For this review, take the finished solid that the model builds, in its own axes (mm). A direction names the side the tool comes from. Give positions to 0.01 mm unless a question says otherwise; leave off trailing zeros. Loops run counter-clockwise (first coordinate to the right, second up) from the corner with the lowest first, then second, coordinate; pieces in that order, holes last.
Autodesk Inventor part; units mm, degrees
ref_plane "YZ Plane" through (0, 0, 0) normal (1, 0, 0) x (0, 1, 0)
ref_plane "XZ Plane" through (0, 0, 0) normal (0, 1, 0) x (-1, 0, 0)
ref_plane "XY Plane" through (0, 0, 0) normal (0, 0, 1) x (1, 0, 0)
sketch "Sketch1" plane through (0, 0, 0) normal (0, 0, 1) x (1, 0, 0)
  circle A0 centre (0, 0) radius 11.5
  arc A1 (20, 0) -> (-20, 0) centre (0, 0) ccw
  line L0 (20, 0) -> (20, -30)
  line L1 (-20, -30) -> (-20, 0)
  line L2 (35, -30) -> (35, -51)
  line L3 (35, -51) -> (-35, -51)
  line L4 (-35, -51) -> (-35, -30)
  line L5 (-35, -30) -> (-20, -30)
  line L6 (20, -30) -> (35, -30)
extrude "Extrusion1" add sketch "Sketch1" along normal blind 6
sketch "Sketch2" plane through (-35, -51, 0) normal (0, -1, 0) x (1, 0, 0)
  line L0 (30, 12) -> (30, -6)
  line L1 (30, -6) -> (40, -6)
  line L2 (40, -6) -> (40, 12)
  line L3 (40, 12) -> (30, 12)
  line L4 (30, 12) -> (40, -6) construction
  line L5 (30, -6) -> (40, 12) construction
  point P0 (35, 0)
  point P1 (35, 3)
  dimension "d7" = 18
  dimension "d8" = 10
extrude "Extrusion2" add sketch "Sketch2" against normal blind 20
fillet "Fillet1" radius 2 6 edges at (5, -41, 6) (-5, -41, 6) (5, -41, 0) (-5, -41, 0) (0, -31, 0) (0, -31, 6)
fillet "Fillet2" radius 4 2 edges at (0, -31, 12) (0, -31, -6)
fillet "Fillet3" radius 4 2 edges at (-35, -30, 3) (35, -30, 3)
sketch "Sketch3" plane through (0, 0, 6) normal (0, 0, 1) x (1, 0, 0)
  arc A0 (7.9976, -11.4908) -> (-7.9976, -11.4908) centre (0, 0) ccw
  arc A1 (7.9976, -16.682) -> (-7.9976, -16.682) centre (0, 0) ccw
  line L0 (4, -12.8417) -> (-4, -19.4934) construction
  line L1 (-4, -12.8417) -> (4, -19.4934) construction
  line L2 (-7.9976, -11.4908) -> (-7.9976, -16.682)
  line L3 (7.9976, -11.4908) -> (7.9976, -16.682)
  point P0 (0, -16.1675)
extrude "Extrusion3" cut sketch "Sketch3" against normal blind 10
sketch "Sketch4" plane through (0, 0, 6) normal (0, 0, 1) x (1, 0, 0)
  line L0 (-7.9976, -11.4908) -> (-7.9976, -16.682)
  line L1 (-7.9976, -16.682) -> (-19.8959, -16.682)
  arc A0 (7.9976, -16.682) -> (-7.9976, -16.682) centre (0, 0) ccw
  line L2 (7.9976, -16.682) -> (20, -16.682)
  line L3 (20, -30) -> (20, 0)
  line L4 (-7.9976, -16.682) -> (-17.0011, 1.4894)
  line L5 (-17.0011, 1.4894) -> (-8.7801, 14.2319)
  line L6 (-8.7801, 14.2319) -> (1.2495, 15.1362)
  line L7 (1.2495, 15.1362) -> (10.7036, 12.5877)
  line L8 (10.7036, 12.5877) -> (15.6744, 3.4985)
  line L9 (15.6744, 3.4985) -> (15.6744, -3.8181)
  line L10 (15.6744, -3.8181) -> (10.5163, -11.3974)
  line L11 (10.5163, -11.3974) -> (8.7045, -14.0594)
  line L12 (8.7045, -14.0594) -> (7.9976, -16.682)
  line L13 (-19.8959, -16.682) -> (-31.3329, 15.1362)
  line L14 (-31.3329, 15.1362) -> (-3.7653, 25.0453)
  line L15 (-3.7653, 25.0453) -> (28.3359, 16.3269)
  line L16 (28.3359, 16.3269) -> (26.8111, -11.3974)
  line L17 (26.8111, -11.3974) -> (20, -16.682)
extrude "Extrusion4" cut sketch "Sketch4" against normal blind 10
sketch "Sketch5" plane through (-19.8959, -16.682, 6) normal (0, 1, 0) x (1, 0, 0)
  line L0 (-7.0101, -7.2709) -> (2.851, -7.2709)
  line L1 (2.851, -7.2709) -> (2.851, 8.3942)
  line L2 (2.851, 8.3942) -> (-7.0101, 8.3942)
  line L3 (-7.0101, 8.3942) -> (-7.0101, -7.2709)
  point P0 (19.8959, 6)
extrude "Extrusion5" cut sketch "Sketch5" along normal blind 10
fillet "Fillet4" radius 10 2 edges at (-20, -16.682, 3) (20, -16.682, 3)
properties part number "Secondary mount"
Q1. Mouldability with a two-part tool opening along Y and no side actions: class faces 6 (the flat face through (25, -30, 3)), 7 (the flat face through (0, -43, -6)), 8 (the cylindrical face through (-17.15, -19.69, 2.96)) as +Y half, -Y half, draft (parallel to the pull), parting line (faces both ways), or undercut.
Answers:
face 6: +Y half
face 7: draft
face 8: undercut
Q2. Machinability: for faces 1 (the flat face through (7.998, -14, 3)), 2 (the flat face through (-20, -28, 3)), 3 (the flat face through (5, -41, 10)), 4 (the cylindrical face through (5.57, -39.85, -0.6)), 5 (the flat face through (-7.998, -14, 3)), which of the approach directions +Z, -Z, +X, -X, +Y, -Y give a long, thin tool a straight path to every point of the face, cutting with its end or side? Answer none if there is none.
Answers:
face 1: +Z, -Z, +X
face 2: +Z, -Z, -X, +Y
face 3: +Z, +X, +Y, -Y
face 4: -Z, +X, +Y, -Y
face 5: +Z, -Z, -X
Q3. For probe 1 along Y at (x, z) = (0, 3.7); probe 2 along X at (y, z) = (-36.5, -3); probe 3 along Z at (x, y) = (7.5, -26.5), list the stretches that pass through material, from the lowest coordinate up.
Answers:
probe 1: y = -51 to -11.5, 11.5 to 14
probe 2: x = -5 to 5
probe 3: z = 0 to 6
Q4. Consider section B-B on y = 0. Give the boundary of the cut face in (x, z), plus the area to 3 significant figures.
Answers:
outline: (-14, 0) - (-11.5, 0) - (-11.5, 6) - (-14, 6) - close; (11.5, 0) - (14, 0) - (14, 6) - (11.5, 6) - close
area: 30.0 mm2
Q5. Consider section D-D on x = -21.5. Give the boundary of the cut face in (y, z).
Answers:
outline: (-51, 0) - (-30, 0) - (-30, 6) - (-51, 6) - close
Q6. Consider section C-C on z = 4.5. Give the boundary of the cut face in (x, y), plus the area to 3 significant figures.
Answers:
outline: (-35, -51) - (35, -51) - (35, -34) arc R4 ccw to (31, -30) - (20, -30) - (20, -26.68) arc R10 ccw to (10, -16.68) - (8, -16.68) - (8, -11.49) arc R14 ccw (long way) to (-8, -11.49) - (-8, -16.68) - (-10, -16.68) arc R10 ccw to (-20, -26.68) - (-20, -30) - (-31, -30) arc R4 ccw to (-35, -34) - close; hole circle Ø23 at (0, 0)
area: 2,210 mm2
Q7. For pin 1 Ø4 at (x, z) = (-4, 1.5) entering from +Y; pin 2 Ø3 at (x, z) = (6.5, 2) entering from +Y; pin 3 Ø1.5 at (x, y) = (21, -39.5) entering from -Z, all flat-tipped, find the tip position at first contact; note any pin that passes through.
Answers:
pin 1: stops at y = 13.86
pin 2: stops at y = 13.08
pin 3: stops at z = 0
